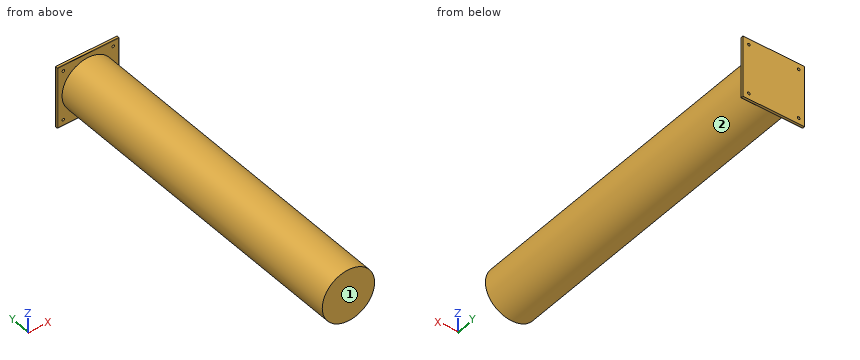
Autodesk Inventor part; units mm, degrees
ref_plane "PlateWorkPlane" through (0, 1020, 0) normal (0, 1, 0) x (1, 0, 0)
ref_plane "YZ Plane" through (0, 0, 0) normal (1, 0, 0) x (0, 1, 0)
ref_plane "XZ Plane" through (0, 0, 0) normal (0, 1, 0) x (-1, 0, 0)
sketch "Sketch1" plane through (0, 0, 0) normal (0, 1, 0) x (-1, 0, 0)
  circle A0 centre (0, 0) radius 80
extrude "InBase" add sketch "Sketch1" along normal blind 400
sketch "Sketch2" plane through (0, 400, 0) normal (0, 1, 0) x (1, 0, 0)
  circle A0 centre (0, 0) radius 80
extrude "AboveBase" add sketch "Sketch2" along normal blind 620
ref_plane "PlateWorkPlane" through (0, 1020, 0) normal (0, 1, 0) x (1, 0, 0)
sketch "Sketch3" plane through (0, 1020, 0) normal (0, 1, 0) x (1, 0, 0)
  line L0 (-94, -94) -> (94, -94)
  line L1 (94, -94) -> (94, 94)
  line L2 (94, 94) -> (-94, 94)
  line L3 (-94, 94) -> (-94, -94)
  line L4 (-94, -94) -> (94, 94) construction
  line L5 (94, -94) -> (-94, 94) construction
  point P0 (0, 0)
extrude "ConnectorPlate" add sketch "Sketch3" along normal blind 8
sketch "Sketch4" plane through (0, 1020, 0) normal (0, -1, 0) x (1, 0, 0)
  point P0 (0, 0)
  point P1 (-76, -76)
  point P2 (-76, 76)
  point P3 (76, 76)
  point P4 (76, -76)
hole "BoltHoles" at (-76, 1020, 76) at (76, 1020, 76) at (76, 1020, -76) at (-76, 1020, -76) direction (0, 1, 0) diameter 8 end through all
fillet "Fillet1" radius 1 4 edges at (0, 1020, 94) (94, 1020, 0) (-94, 1020, 0) (0, 1020, -94)
properties part number "RaAxis"
The model under review builds one solid part; all positions refer to its coordinate system, in mm. Face numbers are marked on the shaded views. A direction names the side the tool comes from. Give positions to 0.01 mm unless a question says otherwise; leave off trailing zeros. Write each loop counter-clockwise with the first axis right and the second up, starting at its lowest first coordinate (ties: lowest second). Pieces come first, ordered by that corner, then holes.
1. Tool access review of the marked faces 1 and 2: name each direction out of +Z, -Z, +X, -X, +Y, -Y from which nothing blocks a thin tool from reaching the whole face with its end or side.
2. For P1, Ø1, axis at y = 837.5, z = -62.5, coming from the +X side; P2, Ø10, axis at x = -69, y = 424.5, coming from the -Z side; P3, Ø6, axis at y = 809.5, z = 23, coming from the -X side; P4, Ø5, axis at x = 76, z = -76, coming from the +Y side, all flat-tipped, find the tip position at first contact; note any pin that passes through.
3. Add section A-A, the plane y = 102.5. Write out the cut boundary in (x, z).
4. Wall thickness on L1, parallel to Z at x = 76, y = 1025; L2, parallel to X at y = 636, z = -4.5: over which ranges is each line inside the solid? List them lowest first.
5. Add section B-B, the plane z = -19.5. Write out the cut boundary in (x, y).
Worked answers:
1. face 1: +Z, -Z, +X, -X, -Y
1. face 2: -Y
2. P1: stops at x = 50.56
2. P2: stops at z = -48
2. P3: stops at x = -77.46
2. P4: passes through
3. outline: circle Ø160 at (0, 0)
4. L1: z = -94 to -80, -72 to 72, 80 to 94
4. L2: x = -79.87 to 79.87
5. outline: (-94, 1021) arc R1 ccw to (-93, 1020) - (-77.59, 1020) - (-77.59, 0) - (77.59, 0) - (77.59, 1020) - (93, 1020) arc R1 ccw to (94, 1021) - (94, 1028) - (-94, 1028) - close
